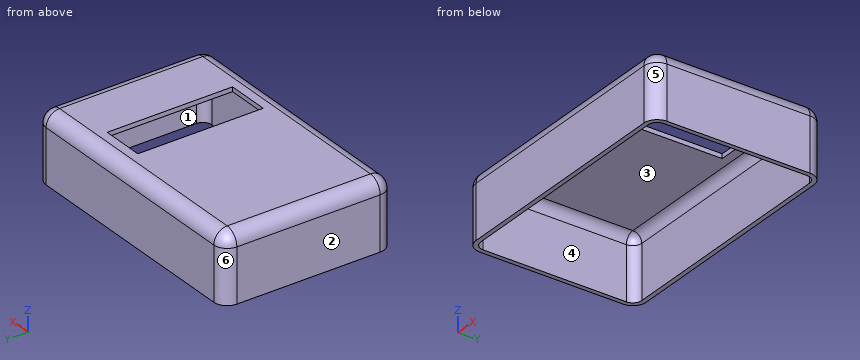
```python
from build123d import *

# Parameters (mm, degrees)
F1_DEPTH = 48.26
F2_R     = 7.62
F3_R     = 7.62
F4_T     = -2.54
F5_W     = 24.13
F5_H     = 71.12
F6_DEPTH = 2.54


with BuildPart() as f1:
    # F0 (on Front) → F1 (new body, symmetric)
    with BuildSketch(Plane.XZ):
        with BuildLine():
            ThreePointArc((73.66, 11.43), (71.4281536726, 16.8181536726), (66.04, 19.05))
            Line((66.04, 19.05), (-66.04, 19.05))
            ThreePointArc((-66.04, 19.05), (-71.4281536726, 16.8181536726), (-73.66, 11.43))
            Line((-73.66, 11.43), (-73.66, -19.05))
            Line((-73.66, -19.05), (73.66, -19.05))
            Line((73.66, -19.05), (73.66, 11.43))
        make_face()
    extrude(amount=F1_DEPTH, both=True)

    # F2
    f2_edges = [f1.edges().sort_by_distance(p)[0] for p in [
        (66.04, 0, 19.05),
        (-66.04, 0, 19.05),
        (71.428154, 48.26, 16.818154),
    ]]
    fillet(f2_edges, radius=F2_R)

    # F3
    f3_edges = [f1.edges().sort_by_distance(p)[0] for p in [
        (66.04, -3.81, 19.05),
        (71.428154, -48.26, 16.818154),
    ]]
    fillet(f3_edges, radius=F3_R)

    # F4
    f4_openings = [f1.faces().sort_by_distance(p)[0] for p in [
        (0, 0, -19.05),
    ]]
    offset(amount=F4_T, openings=f4_openings)

    # F5 (on face) → F6 (cut, through all)
    with BuildSketch(Plane.XY.offset(19.05)):
        with Locations((23.495, 0)):
            Rectangle(F5_W, F5_H)
    extrude(amount=-F6_DEPTH, mode=Mode.SUBTRACT)


solid = f1.part
```
CAD build for the part. Positions are in the model's coordinates, mm. Face numbers are marked on the shaded views. A direction names the side the tool comes from. Round coordinates to 2 decimals unless told otherwise and drop trailing zeros. Loops run counter-clockwise (first coordinate to the right, second up) from the corner with the lowest first, then second, coordinate; pieces in that order, holes last. Notation, with made-up numbers: M 78.5,69.5 L 123.5,69.5 A23 ccw 123.5,79.5 Z; hole C 32,53.5 d5. An arc over 180 degrees is marked long. Return JSON: item names as keys, results as strings. Group by question number.
(1) Tool access for the marked faces 1 and 2: list every direction of +Z, -Z, +X, -X, +Y, -Y with a clear straight run to the whole face (end or side of a thin tool).
(2) Saw through at D-D, the plane z = 14.5. List the corners of the cut face in (x, y).
(3) Mould opens along Y. For the marked faces 3, 4, 5 and 6 say: +Y half, -Y half, draft (parallel to the pull), parting line (faces both ways), or undercut.
(4) Saw through at B-B, the plane z = -15. List the corners of the cut face in (x, y).
(5) Saw through at A-A, the plane y = -11.5. List the corners of the cut face in (x, z), and give its area (3 significant figures).
(6) Drop flat-ended pins along their axis: P1, Ø2, axis at x = -19, y = -15, coming from the -Z side; P2, Ø2, axis at y = 0.5, z = 17.5, coming from the +X side; P3, Ø1.3, axis at x = 28, z = 18, coming from the +Y side; P4, Ø10, axis at x = 18.5, y = 8, coming from the -Z side. Give the stop position or say it passes through.
(7) Saw through at C-C, the plane x = -37.5. List the corners of the cut face in (y, z), and give its area (3 significant figures).
(8) Wall check: probe 1 along Y at (x, z) = (-8, 12); probe 2 along X at (y, z) = (0.5, -2); probe 3 along Y at (x, z) = (35, 10.5). Give the ranges that are in metal, low to high. Write a range as [from, to].
Answer list:
{
 "1": {"face 1": "-Z", "face 2": "+Z, -Z, -X, +Y, -Y"},
 "2": {"outline": "M -73.01,-40.64 A6.97 ccw -66.04,-47.61 L 66.04,-47.61 A6.97 ccw 73.01,-40.64 L 73.01,40.64 A6.97 ccw 66.04,47.61 L -66.04,47.61 A6.97 ccw -73.01,40.64 Z; hole M -70.09,-40.64 A4.05 ccw -66.04,-44.69 L 66.04,-44.69 A4.05 ccw 70.09,-40.64 L 70.09,40.64 A4.05 ccw 66.04,44.69 L -66.04,44.69 A4.05 ccw -70.09,40.64 Z"},
 "3": {"face 3": "undercut", "face 4": "undercut", "face 5": "-Y half", "face 6": "+Y half"},
 "4": {"outline": "M -73.66,-40.64 A7.62 ccw -66.04,-48.26 L 66.04,-48.26 A7.62 ccw 73.66,-40.64 L 73.66,40.64 A7.62 ccw 66.04,48.26 L -66.04,48.26 A7.62 ccw -73.66,40.64 Z; hole M -71.12,-40.64 A5.08 ccw -66.04,-45.72 L 66.04,-45.72 A5.08 ccw 71.12,-40.64 L 71.12,40.64 A5.08 ccw 66.04,45.72 L -66.04,45.72 A5.08 ccw -71.12,40.64 Z"},
 "5": {"outline": "M -73.66,-19.05 L -71.12,-19.05 L -71.12,11.43 A5.08 cw -66.04,16.51 L 11.43,16.51 L 11.43,19.05 L -66.04,19.05 A7.62 ccw -73.66,11.43 Z; M 35.56,16.51 L 66.04,16.51 A5.08 cw 71.12,11.43 L 71.12,-19.05 L 73.66,-19.05 L 73.66,11.43 A7.62 ccw 66.04,19.05 L 35.56,19.05 Z", "area": "480 mm2"},
 "6": {"P1": "z = 16.51", "P2": "x = 71.73", "P3": "y = 45.44", "P4": "through"},
 "7": {"outline": "M -48.26,-19.05 L -45.72,-19.05 L -45.72,11.43 A5.08 cw -40.64,16.51 L 40.64,16.51 A5.08 cw 45.72,11.43 L 45.72,-19.05 L 48.26,-19.05 L 48.26,11.43 A7.62 ccw 40.64,19.05 L -40.64,19.05 A7.62 ccw -48.26,11.43 Z", "area": "412 mm2"},
 "8": {"probe 1": "[-48.24, -45.69], [45.69, 48.24]", "probe 2": "[-73.66, -71.12], [71.12, 73.66]", "probe 3": "[-48.26, -45.72], [45.72, 48.26]"}
}
